Design review of the part built by this model. Coordinates are the model's own, in mm. Face numbers are marked on the shaded views. Round coordinates to 2 decimals unless told otherwise and drop trailing zeros. Loops run counter-clockwise (first coordinate to the right, second up) from the corner with the lowest first, then second, coordinate; pieces in that order, holes last. Notation, with made-up numbers: (1.25, 20.25) - (39.25, 20.25) arc R13 cw to (39.25, 37.25) - close; hole circle Ø9 at (70.5, 6). An arc over 180 degrees is marked (long way). One line per question, with ' | ' between items. Start each with the question number.
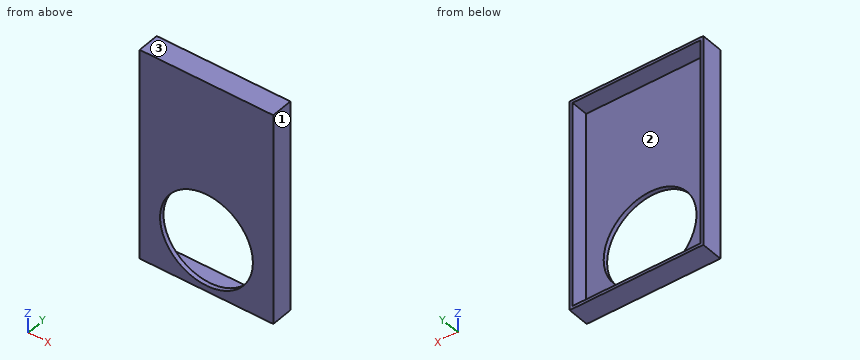
from build123d import *

# Parameters (mm, degrees)
SKETCH1_W           = 61.4
SKETCH1_H           = 48.5
SKETCH1_W_2         = 28.5
SKETCH1_H_2         = 46.5
SKETCH1_W_3         = 28.9
SKETCH1_H_3         = 46.9
BOSS_EXTRUDE1_DEPTH = 35.7
SKETCH2_W           = 29.9
SKETCH2_H           = 48.5
CUT_EXTRUDE1_DEPTH  = 36.7
SKETCH3_W           = 29.2
SKETCH3_H           = 47.2
CUT_EXTRUDE2_DEPTH  = 36.7
SKETCH4_W           = 29.2
SKETCH4_H           = 47.2
SKETCH4_R           = 10.6
BOSS_EXTRUDE2_DEPTH = 1
SKETCH6_W           = 1
SKETCH6_H           = 48.5
CUT_EXTRUDE3_DEPTH  = 36.7
SKETCH7_W           = 30.5
SKETCH7_H           = 30.7
CUT_EXTRUDE4_DEPTH  = 49.5


with BuildPart() as part:
    # Sketch1 → Boss-Extrude1 (new body)
    with BuildSketch(Plane(origin=(0, 0, 0), x_dir=(1, 0, 0), z_dir=(0, 1, 0))):
        with Locations((15.45, -10.593857338)):
            Rectangle(SKETCH1_W, SKETCH1_H)
        with Locations((0, -10.593857338)):
            Rectangle(SKETCH1_W_2, SKETCH1_H_2, mode=Mode.SUBTRACT)
        with Locations((29.7, -10.593857338)):
            Rectangle(SKETCH1_W_3, SKETCH1_H_3, mode=Mode.SUBTRACT)
    extrude(amount=BOSS_EXTRUDE1_DEPTH)

    # Sketch2 → Cut-Extrude1 (cut, through all)
    with BuildSketch(Plane(origin=(0, 35.7, 0), x_dir=(1, 0, 0), z_dir=(0, 1, 0))):
        with Locations((31.2, -10.593857338)):
            Rectangle(SKETCH2_W, SKETCH2_H)
    extrude(amount=-CUT_EXTRUDE1_DEPTH, mode=Mode.SUBTRACT)

    # Sketch3 → Cut-Extrude2 (cut, through all)
    with BuildSketch(Plane(origin=(0, 35.7, 0), x_dir=(1, 0, 0), z_dir=(0, 1, 0))):
        with Locations((0, -10.593857338)):
            Rectangle(SKETCH3_W, SKETCH3_H)
    extrude(amount=-CUT_EXTRUDE2_DEPTH, mode=Mode.SUBTRACT)

    # Sketch4 → Boss-Extrude2 (add)
    with BuildSketch(Plane(origin=(0, 0, 0), x_dir=(1, 0, 0), z_dir=(0, 1, 0))):
        with Locations((0, -10.593857338)):
            Rectangle(SKETCH4_W, SKETCH4_H)
        with Locations((0, 1.756142662)):
            Circle(SKETCH4_R, mode=Mode.SUBTRACT)
    extrude(amount=BOSS_EXTRUDE2_DEPTH)

    # Sketch6 → Cut-Extrude3 (cut, through all)
    with BuildSketch(Plane(origin=(0, 35.7, 0), x_dir=(1, 0, 0), z_dir=(0, 1, 0))):
        with Locations((15.75, -10.593857338)):
            Rectangle(SKETCH6_W, SKETCH6_H)
    extrude(amount=-CUT_EXTRUDE3_DEPTH, mode=Mode.SUBTRACT)

    # Sketch7 → Cut-Extrude4 (cut, through all)
    with BuildSketch(Plane.XY.offset(34.843857338)):
        with Locations((0, 20.35)):
            Rectangle(SKETCH7_W, SKETCH7_H)
    extrude(amount=-CUT_EXTRUDE4_DEPTH, mode=Mode.SUBTRACT)


solid = part.part
1. Take a section at D-D, the plane x = 13.5. Give the boundary of the cut face in (y, z), then the cut area to 3 significant figures.
2. To check wall thickness, follow line 1 along X through (y, z) = (3.8, 23.5); line 2 along Z through (x, y) = (9.5, 3.45); line 3 along Z through (x, y) = (0, 0.4). State the ranges of each line that lie inside material, in increasing order.
3. Take a section at B-B, the plane x = 0. Give the boundary of the cut face in (y, z).
4. Take a section at C-C, the plane z = 3. Give the boundary of the cut face in (x, y).
5. The part is to be moulded in two halves that separate along Z. For the marked faces 1, 2 and 3, say which applies: pulls with the +Z half, pulls with the -Z half, needs draft (parallel to the pull), parting line crosses it, or undercut.
6. Take a section at A-A, the plane y = 1.8. Give the boundary of the cut face in (x, z), then the cut area to 3 significant figures.
7. Clearance check with a flat-ended pin moving along its axis: P1, Ø2, axis at x = 8, z = 19, coming from the +Y side. State where the tip first meets the part, or that it passes through.
Answer list:
1) outline: (0, -13.66) - (5, -13.66) - (5, -13.01) - (1, -13.01) - (1, 34.19) - (5, 34.19) - (5, 34.84) - (0, 34.84) - close | area: 53.7 mm²
2) line 1: x = -15.25 to -14.6, 14.6 to 15.25 | line 2: z = -13.66 to -13.01, 34.19 to 34.84 | line 3: z = -13.66 to -12.36, 8.84 to 34.84
3) outline: (0, -13.66) - (5, -13.66) - (5, -13.01) - (1, -13.01) - (1, -12.36) - (0, -12.36) - close; (0, 8.84) - (1, 8.84) - (1, 34.19) - (5, 34.19) - (5, 34.84) - (0, 34.84) - close
4) outline: (-15.25, 0) - (-9.47, 0) - (-9.47, 1) - (-14.6, 1) - (-14.6, 5) - (-15.25, 5) - close; (9.47, 0) - (15.25, 0) - (15.25, 5) - (14.6, 5) - (14.6, 1) - (9.47, 1) - close
5) face 1: needs draft | face 2: undercut | face 3: pulls with the +Z half
6) outline: (-15.25, -13.66) - (15.25, -13.66) - (15.25, 34.84) - (-15.25, 34.84) - close; hole (-14.6, -13.01) - (14.6, -13.01) - (14.6, 34.19) - (-14.6, 34.19) - close | area: 101 mm²
7) P1: stops at y = 1
